from build123d import *

# Parameters (mm, degrees)
BOSS_EXTRUDE1_DEPTH = 0.254
SKETCH2_R           = 4.699
CUT_EXTRUDE1_DEPTH  = 1.254
SKETCH3_W           = 2.54
SKETCH3_H           = 0.635
CUT_EXTRUDE2_DEPTH  = 1.254
SKETCH5_OUTSIDE_W   = 121.447
SKETCH5_OUTSIDE_H   = 109.618
CUT_EXTRUDE5_DEPTH  = 1.254


with BuildPart() as part:
    # Sketch1 → Boss-Extrude1 (new body)
    with BuildSketch(Plane.XY):
        with BuildLine():
            Line((67.21146711, 76.191723231), (8.696654013, 17.676910134))
            Line((8.696654013, 17.676910134), (7.228954972, 14.133571205))
            ThreePointArc((7.228954972, 14.133571205), (14.666587579, 6.075099489), (15.105587123, -4.88230096))
            Line((15.105587123, -4.88230096), (18.648926052, -6.35))
            Line((18.648926052, -6.35), (101.401368334, -6.35))
            ThreePointArc((101.401368334, -6.35), (93.866160503, 38.880636728), (67.21146711, 76.191723231))
        make_face()
        with BuildLine():
            Line((88.672924278, 6.35), (27.86051193, 6.35))
            ThreePointArc((27.86051193, 6.35), (26.399857642, 10.93517908), (24.190484974, 15.210228852))
            Line((24.190484974, 15.210228852), (67.191354125, 58.211098004))
            ThreePointArc((67.191354125, 58.211098004), (82.13289044, 34.020557137), (88.672924278, 6.35))
        make_face(mode=Mode.SUBTRACT)
    extrude(amount=BOSS_EXTRUDE1_DEPTH)

    # Sketch2 → Cut-Extrude1 (cut, through all)
    with BuildSketch(Plane.XY.offset(0.254)):
        with Locations((22.225, 0)):
            Circle(SKETCH2_R)
        with Locations((36.195, 0)):
            Circle(SKETCH2_R)
        with Locations((61.722, 0)):
            Circle(SKETCH2_R)
        with Locations((75.692, 0)):
            Circle(SKETCH2_R)
        with Locations((95.25, 0)):
            Circle(SKETCH2_R)
        with Locations((15.715448212, 15.715448212)):
            Circle(SKETCH2_R)
        with Locations((25.593729945, 25.593729945)):
            Circle(SKETCH2_R)
        with Locations((43.644044748, 43.644044748)):
            Circle(SKETCH2_R)
        with Locations((53.522326482, 53.522326482)):
            Circle(SKETCH2_R)
        with Locations((92.004434954, 24.652514046)):
            Circle(SKETCH2_R)
        with Locations((82.48891971, 47.625)):
            Circle(SKETCH2_R)
        with Locations((67.351920908, 67.351920908)):
            Circle(SKETCH2_R)
    extrude(amount=-CUT_EXTRUDE1_DEPTH, mode=Mode.SUBTRACT)

    # Sketch3 → Cut-Extrude2 (cut, through all)
    with BuildSketch(Plane.XY.offset(0.254)):
        Polygon((15.266435406, 24.246691527), (17.06248663, 26.042742751), (17.511499436, 25.593729945), (15.715448212, 23.797678721), align=None)
        Polygon((44.991083167, 53.971339288), (43.195031942, 52.175288063), (43.644044748, 51.726275257), (45.440095973, 53.522326482), align=None)
        with Locations((29.21, -6.0325)):
            Rectangle(SKETCH3_W, SKETCH3_H)
        with Locations((68.707, -6.0325)):
            Rectangle(SKETCH3_W, SKETCH3_H)
        Polygon((29.230733674, 38.210989795), (31.026784898, 40.007041019), (31.475797704, 39.558028213), (29.67974648, 37.761976989), align=None)
        Polygon((56.845021246, 65.825277367), (55.048970022, 64.029226143), (55.497982828, 63.580213337), (57.294034052, 65.376264561), align=None)
        with Locations((48.9585, -6.0325)):
            Rectangle(SKETCH3_W, SKETCH3_H)
        with Locations((85.471, -6.0325)):
            Rectangle(SKETCH3_W, SKETCH3_H)
        Polygon((99.935462164, 14.437711971), (100.266998693, 11.919442024), (101.526133667, 12.085210288), (101.194597138, 14.603480236), align=None)
        Polygon((93.765504959, 37.464305742), (94.938831965, 37.950313702), (93.966816047, 40.296967714), (92.793489041, 39.810959755), align=None)
        Polygon((79.327792988, 62.471156422), (80.874047017, 60.456038938), (81.88160576, 61.229165953), (80.33535173, 63.244283437), align=None)
        Polygon((13.593916116, 7.005422516), (14.565932035, 4.658768503), (15.739259041, 5.144776462), (14.767243123, 7.491430475), align=None)
    extrude(amount=-CUT_EXTRUDE2_DEPTH, mode=Mode.SUBTRACT)

    # Sketch5 outside → Cut-Extrude5 (cut, through all)
    with BuildSketch(Plane.XY.offset(0.254)):
        with Locations((54.4145, 34.921)):
            Rectangle(SKETCH5_OUTSIDE_W, SKETCH5_OUTSIDE_H)
        Polygon((30.128759286, 40.905066631), (42.29700633, 53.073313676), (53.073313676, 42.29700633), (40.905066631, 30.128759286), align=None, mode=Mode.SUBTRACT)
    extrude(amount=-CUT_EXTRUDE5_DEPTH, mode=Mode.SUBTRACT)


solid = part.part
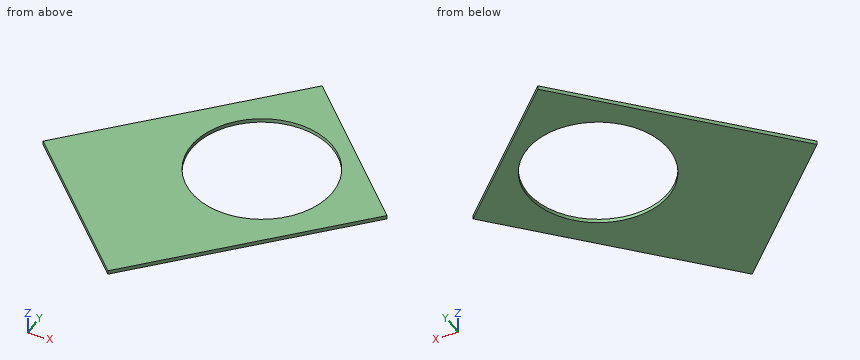
Check sheet for the modelled part. Datum: model origin and axes. Units: mm. Round coordinates to 2 decimals unless told otherwise and drop trailing zeros. Loops run counter-clockwise (first coordinate to the right, second up) from the corner with the lowest first, then second, coordinate; pieces in that order, holes last. Notation, with made-up numbers: M 40.25,79.25 L 57.25,79.25 A14 cw 57.25,88.25 Z; hole C -38.5,23.5 d5. An arc over 180 degrees is marked long. One line per question, with ' | ' between items. Start each with the question number.
Item 1: Scan lines: probe 1 along X at (y, z) = (43, 0.1); probe 2 along X at (y, z) = (41.25, 0.15). Record each from-to range of solid material in increasing order.
Item 2: Section check A-A (x = 42.25). Record the boundary of the cut face in (y, z), and give its area (3 significant figures).
Item 3: Section check C-C (z = 0.15). Record the boundary of the cut face in (x, y).
Item 4: Section check D-D (y = 33). Record the boundary of the cut face in (x, z).
Item 5: Section check B-B (y = 41). Record the boundary of the cut face in (x, z).
Worked out:
1) probe 1: 34.02 to 38.99, 48.3 to 51.98 | probe 2: 32.27 to 39.6, 47.69 to 50.23
2) outline: M 33.27,0 L 39.16,0 L 39.16,0.25 L 33.27,0.25 Z; M 48.13,0 L 51.23,0 L 51.23,0.25 L 48.13,0.25 Z | area: 2.28 mm^2
3) outline: M 31.03,40.01 L 40.01,31.03 L 52.18,43.2 L 43.2,52.18 Z; hole C 43.64,43.64 d9.4
4) outline: M 38.03,0 L 41.98,0 L 41.98,0.25 L 38.03,0.25 Z
5) outline: M 32.02,0 L 39.76,0 L 39.76,0.25 L 32.02,0.25 Z; M 47.53,0 L 49.98,0 L 49.98,0.25 L 47.53,0.25 Z
